Study the drawing (mm; zero at the part's minimum x, y, z) and answer. A direction names the side the tool comes from. Coordinates: 2 decimals unless noted, no trailing zeros. Order: outer loops, then holes, each group sorted by start corner. A loop starts at its lowest first (then second) coordinate and runs counter-clockwise, first axis right, second up. Notation, with made-up numbers: (89, -18) -> (141, -18) arc R37 cw to (141, 21) -> close; hole circle Ø9 at (83, 7). An arc over 180 degrees is marked (long way). One line per question, with ' | ' between items.
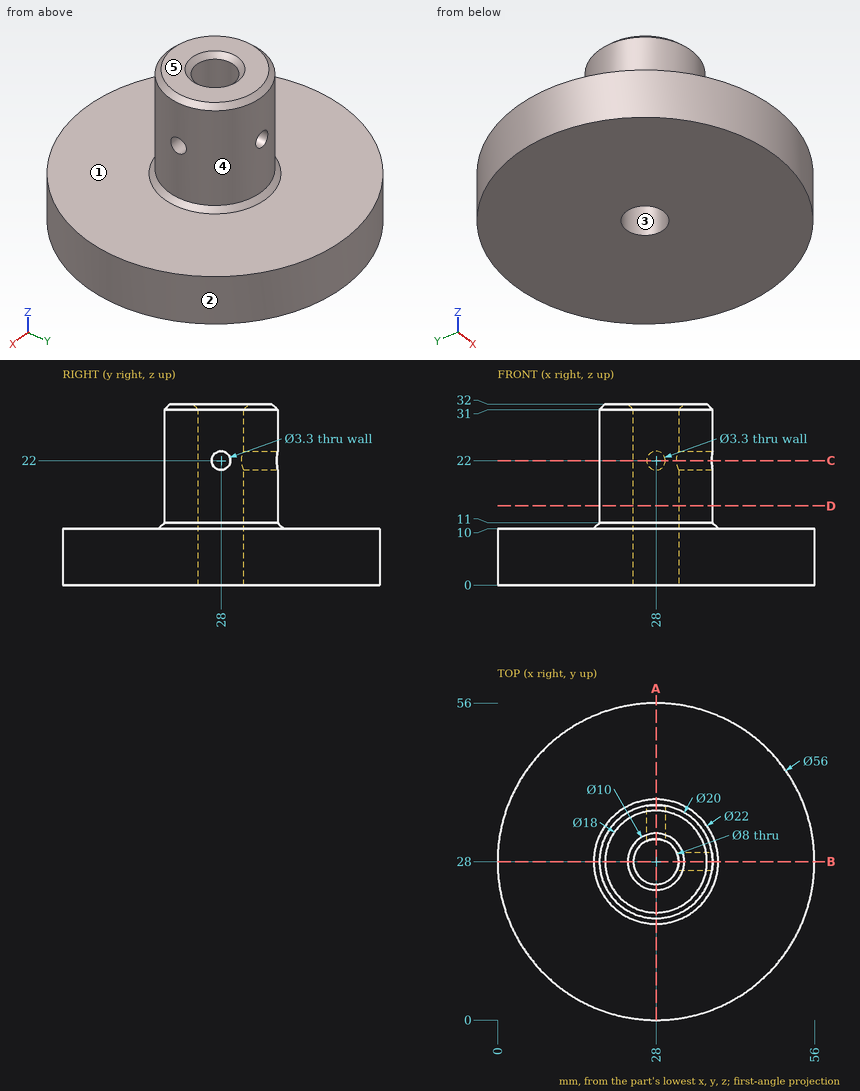
Item 1: Section A-A, the plane x = 28 is taken. Give the vertices of the cut face in (y, z).
Computed values:
outline: (0, 0) -> (24, 0) -> (24, 31) -> (23, 32) -> (19, 32) -> (18, 31) -> (18, 11) -> (17, 10) -> (0, 10) -> close; (32, 0) -> (56, 0) -> (56, 10) -> (39, 10) -> (38, 11) -> (38, 20.35) -> (32, 20.35) -> close; (32, 23.65) -> (38, 23.65) -> (38, 31) -> (37, 32) -> (33, 32) -> (32, 31) -> close
Item 2: Section C-C, the plane z = 22 is taken. Give the vertices of the cut face in (x, y).
Computed values:
outline: (26.35, 31.64) -> (26.35, 37.86) arc R10 ccw (long way) to (37.86, 26.35) -> (31.64, 26.35) arc R4 cw (long way) to start; (29.65, 31.64) arc R4 cw to (31.64, 29.65) -> (37.86, 29.65) arc R10 ccw to (29.65, 37.86) -> close
Item 3: For the marked faces 4 and 5, determine the directions among +Z, -Z, +X, -X, +Y, -Y from which every point of the face is accessible in a straight line to the end or side of a thin tool.
Computed values:
face 4: +Z | face 5: +Z, +X, -X, +Y, -Y
Item 4: Find the intervals of material crossed by L1, parallel to Y at x = 28, z = 7.5; L2, parallel to Z at x = 28, y = 34; L3, parallel to Y at x = 28, z = 15.5, in increasing order.
Computed values:
L1: y = 0 to 24, 32 to 56 | L2: z = 0 to 20.35, 23.65 to 32 | L3: y = 18 to 24, 32 to 38
Item 5: Each of these flat-tipped pins is pushed along its axis until it touches: pin 1 Ø2 at (x, z) = (12, 5.5) entering from +Y; pin 2 Ø1.5 at (x, z) = (29, 9.5) entering from +Y; pin 3 Ø2 at (x, z) = (34.5, 9) entering from +Y. Where does it stop, or does it pass through?
Computed values:
pin 1: stops at y = 51.64 | pin 2: stops at y = 56 | pin 3: stops at y = 55.45
Item 6: Determine the mould class of the marked faces 1, 2 and 3 for opening direction X: pulls with the +X half, pulls with the -X half, needs draft (parallel to the pull), parting line crosses it, or undercut.
Computed values:
face 1: needs draft | face 2: parting line crosses it | face 3: undercut
Item 7: Section D-D, the plane z = 14 is taken. Give the vertices of the cut face in (x, y).
Computed values:
outline: circle Ø20 at (28, 28); hole circle Ø8 at (28, 28)
